Part model, mm, in its own coordinate system. Face numbers are marked on the shaded views. A direction names the side the tool comes from. Coordinates: 2 decimals unless noted, no trailing zeros. Loops run counter-clockwise (first coordinate to the right, second up) from the corner with the lowest first, then second, coordinate; pieces in that order, holes last. Notation, with made-up numbers: (-28.5, 74.5) - (20.5, 74.5) arc R28 ccw to (20.5, 93.5) - close; hole circle Ø3 at (-26, 34.5). An arc over 180 degrees is marked (long way). Use a Markdown table: item, result. Add a question column.
1) Band-saw the part on A-A (x = 0). Give the cut face in (y, z).
2) Tool access for the marked faces 1 and 2: list every direction of +Z, -Z, +X, -X, +Y, -Y with a clear straight run to the whole face (end or side of a thin tool).
3) Drop flat-ended pins along their axis: P1, Ø7, axis at x = -19, y = 0, coming from the +Z side; P2, Ø4, axis at x = -9.5, z = 25, coming from the -Y side; P3, Ø3, axis at y = -7, z = 5, coming from the -X side; P4, Ø5, axis at x = 19, y = 0, coming from the -Z side. Give the stop position or say it passes through.
4) Band-saw the part on C-C (y = 12.5). Give the number of separate pieces and of enclosed holes in the cut face, plus the area to 3 significant figures.
5) Band-saw the part on B-B (z = 26). Give the cut face in (x, y), plus the area to 3 significant figures.
6) Probe probe 1 along X at (y, z) = (12.5, -3.5); probe 2 along Y at (x, z) = (0, 10); probe 3 along X at (y, z) = (-5.5, 30). List the from-to ranges inside material, lowest first. Write a range as [from, to].
Autodesk Inventor part; units mm, degrees
ref_plane "YZ Plane" through (0, 0, 0) normal (1, 0, 0) x (0, 1, 0)
ref_plane "XZ Plane" through (0, 0, 0) normal (0, 1, 0) x (-1, 0, 0)
ref_plane "XY Plane" through (0, 0, 0) normal (0, 0, 1) x (1, 0, 0)
sketch "Szkic1" plane through (0, 0, 0) normal (0, 0, 1) x (1, 0, 0)
  circle A0 centre (0, 0) radius 14
  dimension "d0" = 28
extrude "Wyciągnięcie proste1" add sketch "Szkic1" along normal blind 34
sketch "Szkic2" plane through (0, 0, 0) normal (0, 0, -1) x (-1, 0, 0)
  line L0 (13.2665, -20) -> (-13.2665, -20)
  line L1 (-13.2665, 20) -> (13.2665, 20)
  arc A0 (-13.2665, 20) -> (-13.2665, -20) centre (0, 0) ccw
  arc A1 (13.2665, -20) -> (13.2665, 20) centre (0, 0) ccw
  dimension "d18" = 20
  dimension "d19" = 20
  dimension "d20" = 24
extrude "Wyciągnięcie proste2" add sketch "Szkic2" along normal blind 10
sketch "Szkic3" plane through (0, 0, 34) normal (0, 0, 1) x (1, 0, 0)
  circle A0 centre (0, 0) radius 8
  circle A1 centre (0, 0) radius 11
  dimension "d9" = 16
  dimension "d10" = 3
extrude "Wyciągnięcie proste3" cut sketch "Szkic3" against normal up to surface (44 mm away) contours A0
extrude "Wyciągnięcie proste4" cut sketch "Szkic3" against normal blind 0.5
sketch "Szkic4" plane through (0, 0, -10) normal (0, 0, -1) x (-1, 0, 0)
  circle A0 centre (0, 0) radius 8
  circle A1 centre (0, 0) radius 11
  circle A2 centre (0, 0) radius 19
  line L0 (-13.435, -13.435) -> (0, 0)
  line L1 (0, 0) -> (13.435, 13.435)
  line L2 (0, 0) -> (13.435, -13.435)
  line L3 (0, 0) -> (-13.435, 13.435)
  line L4 (-27.1999, 0) -> (26.3201, 0)
  arc A3 (-13.2665, 20) -> (-13.2665, -20) centre (0, 0) ccw
  line L5 (-13.2665, -20) -> (13.2665, -20)
  arc A4 (13.2665, -20) -> (13.2665, 20) centre (0, 0) ccw
  line L6 (13.2665, 20) -> (-13.2665, 20)
  point P0 (-19, 0)
  point P1 (19, 0)
  dimension "d15" = 3
  dimension "d23" = 19
  dimension "d28" = 38
  dimension "d29" = 45
  dimension "d30" = 45
  dimension "d31" = 45
  dimension "d32" = 45
extrude "Wyciągnięcie proste5" cut sketch "Szkic4" against normal blind 0.5 contours L4 A1 L2 A0 | A0 L1 A1 L4 | A0 L3 A1 L1 | L2 A1 L0 A0 | A0 L4 A1 L3 | L0 A1 L4 A0
hole "Otwór1" at (13.435, -13.435, -10) at (19, 0, -10) at (13.435, 13.435, -10) at (-13.435, 13.435, -10) at (-19, 0, -10) at (-13.435, -13.435, -10) direction (0, 0, 1) diameter 5.5 end through all
chamfer "Faza1" distance 1 angle 45 4 edges at (-24, 0, 0) (-24, 0, -10) (24, 0, 0) (24, 0, -10)
chamfer "Faza2" distance 0.6 angle 45 1 edges at (-14, 0, 34)
properties part number "COTS_GENERIC_SFU1605_Ball_Screw_Nut"
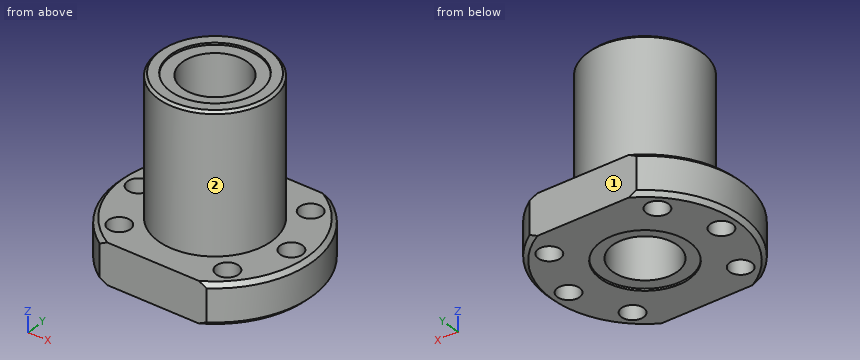
Answer block:
| question | item | result |
|---|---|---|
| 1 | outline | (-20, -10) - (-11, -10) - (-11, -9.5) - (-8, -9.5) - (-8, 33.5) - (-11, 33.5) - (-11, 34) - (-13.4, 34) - (-14, 33.4) - (-14, 0) - (-20, 0) - close; (8, -9.5) - (11, -9.5) - (11, -10) - (20, -10) - (20, 0) - (14, 0) - (14, 33.4) - (13.4, 34) - (11, 34) - (11, 33.5) - (8, 33.5) - close |
| 2 | face 1 | +Z, -Z, +X, -X, +Y |
| 2 | face 2 | +Z |
| 3 | P1 | z = 0 |
| 3 | P2 | y = -11.82 |
| 3 | P3 | x = -12.87 |
| 3 | P4 | through |
| 4 | separate pieces | 3 |
| 4 | enclosed holes | 0 |
| 4 | area | 732 mm2 |
| 5 | outline | circle Ø28 at (0, 0); hole circle Ø16 at (0, 0) |
| 5 | area | 415 mm2 |
| 6 | probe 1 | [-20.49, -16.02], [-10.85, 10.85], [16.02, 20.49] |
| 6 | probe 2 | [-14, -8], [8, 14] |
| 6 | probe 3 | [-12.87, -5.81], [5.81, 12.87] |
